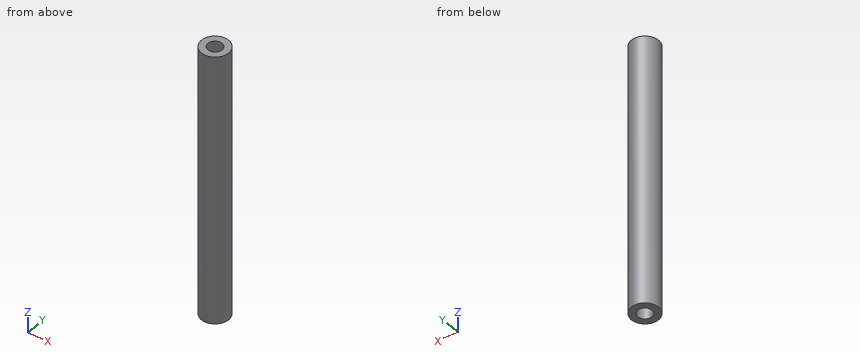
from build123d import *

# Parameters (mm, degrees)
SKETCH1_R                 = 2.5
BOSS_EXTRUDE1_DEPTH       = 49.5
M3X0_5_TAPPED_HOLE1_D     = 2.6
M3X0_5_TAPPED_HOLE1_DEPTH = 8
M3X0_5_TAPPED_HOLE1_TIP   = 0.781118805
M3X0_5_TAPPED_HOLE2_D     = 2.6
M3X0_5_TAPPED_HOLE2_DEPTH = 8
M3X0_5_TAPPED_HOLE2_TIP   = 0.781118805


with BuildPart() as part:
    # Sketch1 → Boss-Extrude1 (new body)
    with BuildSketch(Plane.XY):
        Circle(SKETCH1_R)
    extrude(amount=BOSS_EXTRUDE1_DEPTH)

    # M3x0.5 Tapped Hole1
    with Locations(Plane.XY.offset(49.5)):
        with Locations((0, 0)):
            Hole(M3X0_5_TAPPED_HOLE1_D / 2, depth=M3X0_5_TAPPED_HOLE1_DEPTH)
            with Locations((0, 0, -(M3X0_5_TAPPED_HOLE1_DEPTH + M3X0_5_TAPPED_HOLE1_TIP / 2))):  # 118° drill point
                Cone(0, M3X0_5_TAPPED_HOLE1_D / 2, M3X0_5_TAPPED_HOLE1_TIP, mode=Mode.SUBTRACT)

    # M3x0.5 Tapped Hole2
    with Locations(Plane(origin=(0, 0, 0), x_dir=(-1, 0, 0), z_dir=(0, 0, -1))):
        with Locations((0, 0)):
            Hole(M3X0_5_TAPPED_HOLE2_D / 2, depth=M3X0_5_TAPPED_HOLE2_DEPTH)
            with Locations((0, 0, -(M3X0_5_TAPPED_HOLE2_DEPTH + M3X0_5_TAPPED_HOLE2_TIP / 2))):  # 118° drill point
                Cone(0, M3X0_5_TAPPED_HOLE2_D / 2, M3X0_5_TAPPED_HOLE2_TIP, mode=Mode.SUBTRACT)


solid = part.part
Could you check a few things on this model? Use its own coordinates, in mm. Coordinates: 2 decimals unless noted, no trailing zeros. Order: outer loops, then holes, each group sorted by start corner. A loop starts at its lowest first (then second) coordinate and runs counter-clockwise, first axis right, second up. Notation, with made-up numbers: (-5, 71.25) -> (50, 71.25) arc R19 cw to (50, 101.25) -> close; hole circle Ø9 at (3.5, 63). An arc over 180 degrees is marked (long way). One line per question, with ' | ' between items.
Q1. Imagine slicing it at A-A on z = 13. Please give me the cut outline in (x, y).
Return value:
outline: circle Ø5 at (0, 0)
Q2. Imagine slicing it at B-B on x = -1.75. Please give me the cut outline in (y, z).
Return value:
outline: (-1.79, 0) -> (1.79, 0) -> (1.79, 49.5) -> (-1.79, 49.5) -> close
Q3. If I drill on L1, parallel to Y at x = 0, z = 46.5; L2, parallel to X at y = -0.1, z = 37; L3, parallel to X at y = 0.95, z = 3.5, over which ranges is the centre line in solid material (lowest first)?
Return value:
L1: -2.5 to -1.3, 1.3 to 2.5 | L2: -2.5 to 2.5 | L3: -2.31 to -0.89, 0.89 to 2.31
Q4. I'm going to push flat-ended pins straight in: P1, Ø2, axis at x = 0, y = 0, coming from the -Z side; P2, Ø1.5, axis at x = -1, z = 5, coming from the -Y side; P3, Ø1, axis at y = -1, z = 8.5, coming from the +X side; P4, Ø3, axis at x = 0, y = 0, coming from the -Z side. Where does each tip first touch, or does it pass through?
Return value:
P1: z = 8.18 | P2: y = -2.49 | P3: x = 2.45 | P4: z = 0
